```python
from build123d import *

# Parameters (mm, degrees)
F0_W     = 15.875
F0_H     = 7.9375
F1_DEPTH = 9.525
F2_R     = 2.4257
F4_DEPTH = 1.778
F3_R     = 2.4257
F5_DEPTH = 1.778
F6_W     = 13.6906
F6_H     = 5.7531
F7_DEPTH = 8.4328


with BuildPart() as f1:
    # F0 (on Top) → F1 (new body)
    with BuildSketch(Plane.XY):
        with Locations((-20.961086, 23.913214)):
            Rectangle(F0_W, F0_H)
    extrude(amount=F1_DEPTH)

    # F2 (on face) → F4 (join)
    with BuildSketch(Plane.XY.offset(9.525)):
        with Locations((-24.936186, 23.919564)):
            Circle(F2_R)
    extrude(amount=F4_DEPTH)

    # F3 (on face) → F5 (join)
    with BuildSketch(Plane.XY.offset(9.525)):
        with Locations((-16.985986, 23.919564)):
            Circle(F3_R)
    extrude(amount=F5_DEPTH)

    # F6 (on face) → F7 (cut)
    with BuildSketch(Plane(origin=(0, 0, 0), x_dir=(1, 0, 0), z_dir=(0, 0, -1))):
        with Locations((-20.961086, -23.913214)):
            Rectangle(F6_W, F6_H)
    extrude(amount=-F7_DEPTH, mode=Mode.SUBTRACT)


solid = f1.part
```
Could you check a few things on this model? Use its own coordinates, in mm. A direction names the side the tool comes from. Give positions to 0.01 mm unless a question says otherwise; leave off trailing zeros. Order: outer loops, then holes, each group sorted by start corner. A loop starts at its lowest first (then second) coordinate and runs counter-clockwise, first axis right, second up.
Q1. Suppose I cut it at B-B, the plane z = 5. Write out the boundary of the cut face in (x, y).
Q2. Suppose I cut it at A-A, the plane x = -20. Write out the boundary of the cut face in (y, z) (3 decimals).
Q3. I'm going to push flat-ended pins straight in: P1, Ø3, axis at x = -22, y = 23, coming from the -Z side; P2, Ø4, axis at y = 26.5, z = 10, coming from the -X side. Where does each tip first touch, or does it pass through?
Q4. Suppose I cut it at C-C, the plane y = 24.25. Write out the boundary of the cut face in (x, z) (3 decimals).
Q5. We'd pull the mould along X, two halves only. Please class faces 4 (the flat face through (-13.024, 24, 5)), 5 (the flat face through (-14.116, 24, 4)), 6 (the flat face through (-21, 19.944, 5)): +X half, -X half, draft (parallel to the pull), parting line (faces both ways), or undercut.
Q6. If I drill on line 1 along X through (y, z) = (26, 5.25); line 2 along Y through (x, z) = (-18, 7.75); line 3 along Z through (x, y) = (-27, 26) (3 decimals), over which ranges is the centre line in solid material (lowest first)?
Q7. For faces 1 (the flat face through (-25, 24, 11.303)), 2 (the cylindrical face through (-18.91, 22.44, 10.4)), 3 (the flat face through (-21, 21.037, 4)), which set-ups out of +Z, -Z, +X, -X, +Y, -Y let a thin tool reach every point of the face, with its end or its side?
Q8. Suppose I cut it at D-D, the plane z = 10.5. Write out the boundary of the cut face in (x, y), and give its area (3 significant figures).
Solution:
1. outline: (-28.9, 19.94) - (-13.02, 19.94) - (-13.02, 27.88) - (-28.9, 27.88) - close; hole (-27.81, 21.04) - (-14.12, 21.04) - (-14.12, 26.79) - (-27.81, 26.79) - close
2. outline: (19.944, 0) - (21.037, 0) - (21.037, 8.433) - (26.79, 8.433) - (26.79, 0) - (27.882, 0) - (27.882, 9.525) - (19.944, 9.525) - close
3. P1: stops at z = 8.43
3. P2: stops at x = -28.9
4. outline: (-28.899, 0) - (-27.806, 0) - (-27.806, 8.433) - (-14.116, 8.433) - (-14.116, 0) - (-13.024, 0) - (-13.024, 9.525) - (-14.583, 9.525) - (-14.583, 11.303) - (-19.389, 11.303) - (-19.389, 9.525) - (-22.533, 9.525) - (-22.533, 11.303) - (-27.339, 11.303) - (-27.339, 9.525) - (-28.899, 9.525) - close
5. face 4: +X half
5. face 5: undercut
5. face 6: draft
6. line 1: x = -28.9 to -27.81, -14.12 to -13.02
6. line 2: y = 19.94 to 21.04, 26.79 to 27.88
6. line 3: z = 8.433 to 9.525
7. face 1: +Z, +X, -X, +Y, -Y
7. face 2: +Z
7. face 3: -Z
8. outline: circle Ø4.85 at (-24.94, 23.92); circle Ø4.85 at (-16.99, 23.92)
8. area: 37.0 mm2
